Input: dimensioned drawing with shaded views. Units: mm. Origin: part minimum x, y, z. Give positions to 0.01 mm unless a question says otherwise; leave off trailing zeros. Loops run counter-clockwise (first coordinate to the right, second up) from the corner with the lowest first, then second, coordinate; pieces in that order, holes last. Notation, with made-up numbers: M -10.75,11.25 L 18.25,11.25 A28 cw 18.25,49.25 Z; hole C 4.25,8 d11. An arc over 180 degrees is marked long. Answer in a Markdown table with one row per item.
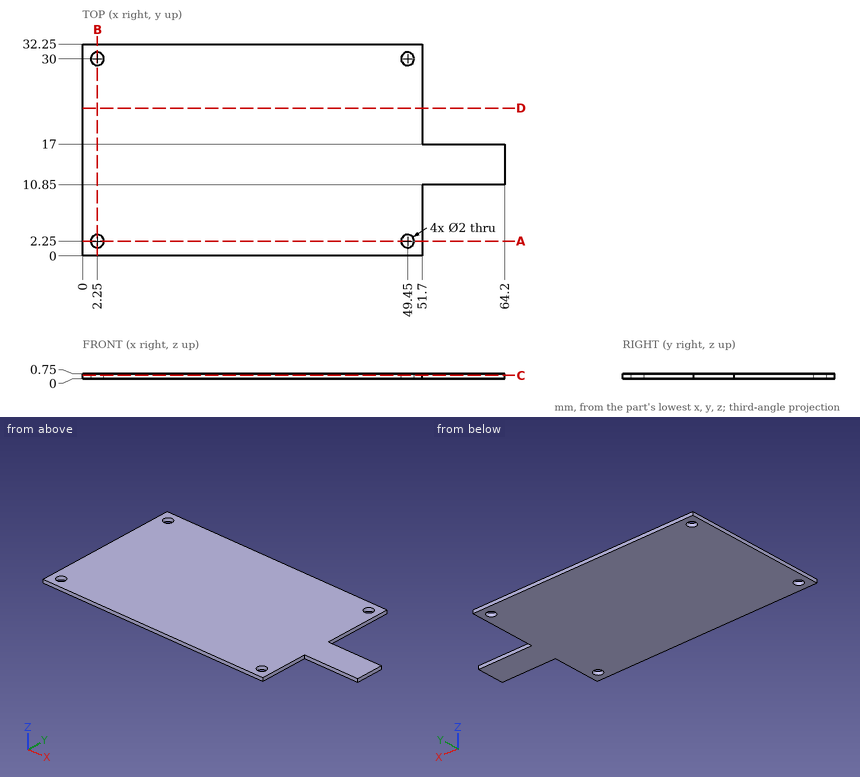
Q1. Section query A-A (y = 2.25). Output: boundary loops of the cut face in (x, z).
Values follow:
| item | result |
|---|---|
| outline | M 0,0 L 1.25,0 L 1.25,0.75 L 0,0.75 Z; M 3.25,0 L 48.45,0 L 48.45,0.75 L 3.25,0.75 Z; M 50.45,0 L 51.7,0 L 51.7,0.75 L 50.45,0.75 Z |
Q2. Section query C-C (z = 0.55). Output: boundary loops of the cut face in (x, y).
Values follow:
| item | result |
|---|---|
| outline | M 0,0 L 51.7,0 L 51.7,10.85 L 64.2,10.85 L 64.2,17 L 51.7,17 L 51.7,32.25 L 0,32.25 Z; hole C 2.25,2.25 d2; hole C 2.25,30 d2; hole C 49.45,2.25 d2; hole C 49.45,30 d2 |
Q3. Section query B-B (x = 2.25). Output: boundary loops of the cut face in (y, z).
Values follow:
| item | result |
|---|---|
| outline | M 0,0 L 1.25,0 L 1.25,0.75 L 0,0.75 Z; M 3.25,0 L 29,0 L 29,0.75 L 3.25,0.75 Z; M 31,0 L 32.25,0 L 32.25,0.75 L 31,0.75 Z |
Q4. Ray query, probe 1 along Y at (x, z) = (49.45, 0.45); probe 2 along Y at (x, z) = (3, 0.6); probe 3 along X at (y, z) = (19, 0.55). Return the intervals inside material, ascending. Write a range as from..to.
Values follow:
| item | result |
|---|---|
| probe 1 | 0..1.25, 3.25..29, 31..32.25 |
| probe 2 | 0..1.59, 2.91..29.34, 30.66..32.25 |
| probe 3 | 0..51.7 |
Q5. Section query D-D (y = 22.5). Output: boundary loops of the cut face in (x, z), plus the area to 3 significant figures.
Values follow:
| item | result |
|---|---|
| outline | M 0,0 L 51.7,0 L 51.7,0.75 L 0,0.75 Z |
| area | 38.8 mm^2 |
